from build123d import *

# Parameters (mm, degrees)
SKETCH1_W               = 92
SKETCH1_H               = 70
SKETCH1_R               = 14
BOSS_EXTRUDE1_DEPTH     = 5
CUT_EXTRUDE1_DEPTH      = 116.71084651
CUT_EXTRUDE1_DEPTH_BACK = 116.71084651
SKETCH2_R               = 2.5


with BuildPart() as part:
    # Sketch1 → Boss-Extrude1 (new body)
    with BuildSketch(Plane(origin=(0, 0, 0), x_dir=(0, 0, -1), z_dir=(1, 0, 0))):
        with Locations((46, -35)):
            Rectangle(SKETCH1_W, SKETCH1_H)
        with Locations((46, -35)):
            Circle(SKETCH1_R, mode=Mode.SUBTRACT)
    extrude(amount=BOSS_EXTRUDE1_DEPTH)

    # Sketch2 → Cut-Extrude1 (cut, two sides: drawn at the far end of the back side and taken through both)
    with BuildSketch(Plane(origin=(5, 0, 0), x_dir=(0, 0, -1), z_dir=(1, 0, 0)).offset(-CUT_EXTRUDE1_DEPTH_BACK)):
        with Locations((5, -16.272445859)):
            Circle(SKETCH2_R)
        with Locations((5, -53.727554141)):
            Circle(SKETCH2_R)
        with Locations((87, -53.727554141)):
            Circle(SKETCH2_R)
        with Locations((87, -16.272445859)):
            Circle(SKETCH2_R)
    extrude(amount=CUT_EXTRUDE1_DEPTH + CUT_EXTRUDE1_DEPTH_BACK, mode=Mode.SUBTRACT)


solid = part.part
The listing builds one solid part. Answer for the finished solid, in the listing's coordinates (mm). Coordinates: 2 decimals unless noted, no trailing zeros. Write each loop counter-clockwise with the first axis right and the second up, starting at its lowest first coordinate (ties: lowest second). Pieces come first, ordered by that corner, then holes. Notation, with made-up numbers: M 71.5,38 L 79.5,38 A27 cw 79.5,59 Z; hole C 36.25,-11.75 d2. An arc over 180 degrees is marked long. Put each result on its own line as item: value. Start each with the question number.
1. Consider line 1 (Y direction, x = 2.9, z = -5); line 2 (Y direction, x = 2.7, z = -46); line 3 (Z direction, x = 3.1, y = -54.5). Determine where each line is inside the solid, lowest interval first. Write a range as from..to.
2. Flat-ended cylindrical pins translate along their axes: P1, Ø6, axis at y = -26.5, z = -57, coming from the +X side; P2, Ø3, axis at y = -16.27, z = -87, coming from the -X side. Find the tip coordinate at first contact, or state that the pin passes through.
3. A cutting plane is placed at B-B on y = -35. Write down the section's boundary in (x, z).
4. For a pull along Z with two mould halves and no side action, classify faces 1 (the flat face through (0, -50, -45)), 2 (the flat face through (2, -35, 0)), 3 (the cylindrical face through (2.465, -55.249, -85.016)) as pulls with the +Z half, pulls with the -Z half, needs draft (parallel to the pull), parting line crosses it, or undercut.
5. A cutting plane is placed at D-D on z = -40. Write down the section's boundary in (x, y).
6. A cutting plane is placed at A-A on z = -5. Write down the section's boundary in (x, y).
7. A cutting plane is placed at C-C on x = 3.3. Write down the section's boundary in (y, z).
Resolved:
1. line 1: y = -70..-56.23, -51.23..-18.77, -13.77..0
1. line 2: y = -70..-49, -21..0
1. line 3: z = -92..-89.38, -84.62..-7.38, -2.62..0
2. P1: stops at x = 5
2. P2: passes through
3. outline: M 0,-92 L 5,-92 L 5,-60 L 0,-60 Z; M 0,-32 L 5,-32 L 5,0 L 0,0 Z
4. face 1: needs draft
4. face 2: pulls with the +Z half
4. face 3: undercut
5. outline: M 0,-70 L 5,-70 L 5,-47.65 L 0,-47.65 Z; M 0,-22.35 L 5,-22.35 L 5,0 L 0,0 Z
6. outline: M 0,-70 L 5,-70 L 5,-56.23 L 0,-56.23 Z; M 0,-51.23 L 5,-51.23 L 5,-18.77 L 0,-18.77 Z; M 0,-13.77 L 5,-13.77 L 5,0 L 0,0 Z
7. outline: M -70,-92 L 0,-92 L 0,0 L -70,0 Z; hole C -53.73,-87 d5; hole C -53.73,-5 d5; hole C -35,-46 d28; hole C -16.27,-87 d5; hole C -16.27,-5 d5
